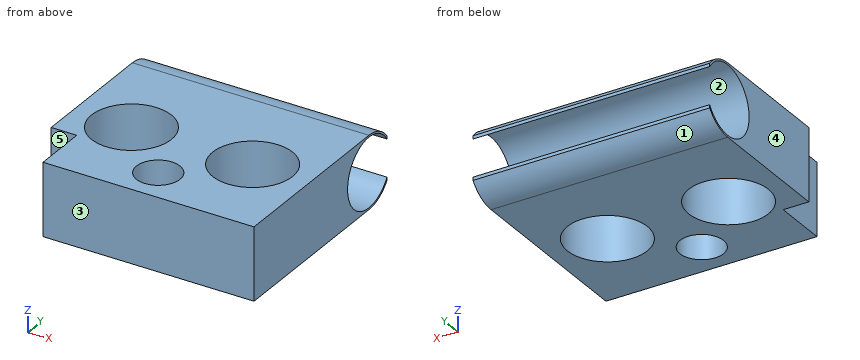
from build123d import *

# Parameters (mm, degrees)
PARALLELEPIPEDOBLOCCO_DEPTH      = 20
SCHIZZO2_R                       = 11
SCHIZZO2_R_2                     = 6
FORITUBIMOTORI_DEPTH             = 54.183667606
SCHIZZO4_R                       = 9.5
FOROLONGHERONE_DEPTH             = 78.504903071
ELIMINAZIONEPARTESUPERIORE_DEPTH = 78.504903071
SCHIZZO6_W                       = 7.05
SCHIZZO6_H                       = 15
SPAZIOMOVIMENTOLEVETTA_DEPTH     = 53.49288047
SCHIZZO7_W                       = 20
SCHIZZO7_H                       = 2
RIMOZIONEPARTESUPERIORE_DEPTH    = 65.1


with BuildPart() as part:
    # Schizzo1 → ParallelepipedoBlocco (new body)
    with BuildSketch(Plane.XY):
        Polygon((-30.55, -25), (30.55, -25), (32.55, -25), (32.55, 17), (32.55, 37), (-32.55, 37), (-32.55, 17), (-32.55, -25), align=None)
    extrude(amount=PARALLELEPIPEDOBLOCCO_DEPTH)

    # Schizzo2 → ForiTubiMotori (cut, through all)
    with BuildSketch(Plane.XY.offset(20)):
        with Locations((-16.665, 0)):
            Circle(SCHIZZO2_R)
        with Locations((16.665, 0)):
            Circle(SCHIZZO2_R)
        with Locations((0, -15)):
            Circle(SCHIZZO2_R_2)
    extrude(amount=-FORITUBIMOTORI_DEPTH, mode=Mode.SUBTRACT)

    # Schizzo4 → ForoLongherone (cut, through all)
    with BuildSketch(Plane.ZY.offset(32.55)):
        with Locations((10, 26)):
            Circle(SCHIZZO4_R)
    extrude(amount=-FOROLONGHERONE_DEPTH, mode=Mode.SUBTRACT)

    # Schizzo5 → EliminazioneParteSuperiore (cut, through all)
    with BuildSketch(Plane.ZY.offset(32.55)):
        with BuildLine():
            Line((0, 26), (0, 37))
            Line((0, 37), (20, 37))
            Line((20, 37), (20, 26))
            ThreePointArc((20, 26), (10, 36), (0, 26))
        make_face()
    extrude(amount=-ELIMINAZIONEPARTESUPERIORE_DEPTH, mode=Mode.SUBTRACT)

    # Schizzo6 → SpazioMovimentoLevetta (cut, through all)
    with BuildSketch(Plane.XY.offset(20)):
        with Locations((-29.025, -17.5)):
            Rectangle(SCHIZZO6_W, SCHIZZO6_H)
    extrude(amount=-SPAZIOMOVIMENTOLEVETTA_DEPTH, mode=Mode.SUBTRACT)

    # Schizzo7 → RimozioneParteSuperiore (cut)
    with BuildSketch(Plane.ZY.offset(32.55)):
        with Locations((10, 35)):
            Rectangle(SCHIZZO7_W, SCHIZZO7_H)
    extrude(amount=-RIMOZIONEPARTESUPERIORE_DEPTH, mode=Mode.SUBTRACT)


solid = part.part
For this review, take the finished solid that the model builds, in its own axes (mm). Face numbers are marked on the shaded views. A direction names the side the tool comes from. Round coordinates to 2 decimals unless told otherwise and drop trailing zeros. Loops run counter-clockwise (first coordinate to the right, second up) from the corner with the lowest first, then second, coordinate; pieces in that order, holes last. Notation, with made-up numbers: (0.25, 29.5) - (23.25, 29.5) arc R13 cw to (23.25, 49.5) - close; hole circle Ø1 at (85.25, 16). An arc over 180 degrees is marked (long way). Put each result on its own line as item: value. Start each with the question number.
1. For probe 1 along Z at (x, y) = (11, 26); probe 2 along Y at (x, z) = (-25, 4.5); probe 3 along Y at (x, z) = (2, 17.5), list the stretches that pass through material, from the lowest coordinate up. Write a range as [from, to].
2. Consider section D-D on y = 0. State the section outline as (x, z) points (3 decimals).
3. Consider section B-B on y = -15. State the section outline as (x, z) points, plus the area to 3 significant figures.
4. Consider section C-C on z = 10. State the section outline as (x, y) points (3 decimals), plus the area to 3 significant figures.
5. Consider section A-A on x = 0. State the section outline as (y, z) points, plus the area to 3 significant figures.
6. For the marked faces 4 and 5, list the 3-axis set-ups (+Z, -Z, +X, -X, +Y, -Y) from which the entire face can be reached by the end or side of a thin tool; tool diameter is ignored.
7. Insertion check: P1, Ø1.5, axis at x = 9, z = 12.5, coming from the +Y side. The pin has a flat end and moves straight along its axis. Give the tip position at first contact, or say it passes through.
8. Mouldability with a two-part tool opening along Z and no side actions: class the marked faces 1, 2 and 3 as +Z half, -Z half, draft (parallel to the pull), parting line (faces both ways), or undercut.
Result sheet:
1. probe 1: [0, 0.5], [19.5, 20]
1. probe 2: [-25, -7.18], [7.18, 18.25], [33.75, 34]
1. probe 3: [-25, -20.66], [-9.34, 20.17], [31.83, 32.61]
2. outline: (-32.55, 0) - (-27.665, 0) - (-27.665, 20) - (-32.55, 20) - close; (-5.665, 0) - (5.665, 0) - (5.665, 20) - (-5.665, 20) - close; (27.665, 0) - (32.55, 0) - (32.55, 20) - (27.665, 20) - close
3. outline: (-25.5, 0) - (-6, 0) - (-6, 20) - (-25.5, 20) - close; (6, 0) - (32.55, 0) - (32.55, 20) - (6, 20) - close
3. area: 921 mm^2
4. outline: (-32.55, -10) - (-25.5, -10) - (-25.5, -25) - (32.55, -25) - (32.55, 16.5) - (-32.55, 16.5) - close; hole circle Ø22 at (-16.665, 0); hole circle Ø12 at (0, -15); hole circle Ø22 at (16.665, 0)
4. area: 1,720 mm^2
5. outline: (-25, 0) - (-21, 0) - (-21, 20) - (-25, 20) - close; (-9, 0) - (26, 0) arc R10 ccw to (34, 4) - (34, 4.88) arc R9.5 cw (long way) to (34, 15.12) - (34, 16) arc R10 ccw to (26, 20) - (-9, 20) - close
5. area: 648 mm^2
6. face 4: +Z, -Z, -X, +Y, -Y
6. face 5: +Z, -Z, -X, -Y
7. P1: y = 17.07
8. face 1: -Z half
8. face 2: undercut
8. face 3: draft
